Autodesk Inventor part; units mm, degrees
ref_plane "YZ Plane" through (0, 0, 0) normal (1, 0, 0) x (0, 1, 0)
ref_plane "XZ Plane" through (0, 0, 0) normal (0, 1, 0) x (-1, 0, 0)
ref_plane "XY Plane" through (0, 0, 0) normal (0, 0, 1) x (1, 0, 0)
sketch "スケッチ1" plane through (0, 0, 0) normal (1, 0, 0) x (0, 1, 0)
  line L0 (-5, 30) -> (5, 30)
  line L1 (5, 30) -> (5, 0)
  line L2 (5, 0) -> (-5, 0)
  line L3 (-5, 0) -> (-5, 30)
  line L4 (-15, 45) -> (15, 45)
  line L5 (15, 45) -> (15, 30)
  line L6 (15, 30) -> (-15, 30)
  line L7 (-15, 30) -> (-15, 45)
  line L8 (15, 30) -> (5, 0)
  line L9 (-5, 0) -> (-15, 30)
  point P0 (0, 0)
  point P1 (0, 0)
  point P2 (0, 30)
  dimension "d0" = 10
  dimension "d1" = 30
  dimension "d2" = 30
  dimension "d3" = 15
extrude "押し出し1" add sketch "スケッチ1" along normal blind 2
sketch "スケッチ2" plane through (2, 0, 0) normal (1, 0, 0) x (0, 0, -1)
  line L0 (0, -5) -> (0, 5)
  line L1 (-30, 15) -> (-45, 15)
  line L2 (-45, -15) -> (-30, -15)
  point P0 (0, 0)
  point P1 (-37.5, 10)
  point P2 (-37.5, -10)
  point P3 (-25, 0)
  point P4 (-5, 0)
  point P5 (0, 0)
  point P6 (-37.5, 15)
  dimension "d6" = 5
  dimension "d7" = 20
  dimension "d8" = 5
  dimension "d9" = 5
hole "穴1" at (2, 10, 37.5) at (2, -10, 37.5) at (2, 0, 25) at (2, 0, 5) direction (-1, 0, 0) diameter 3.2 end through all
properties part number "FrameJointT1510" material "アルミニウム 6061"
Work out the finished part from the listing and answer in its coordinate system (mm). Give positions to 0.01 mm unless a question says otherwise; leave off trailing zeros. Loops run counter-clockwise (first coordinate to the right, second up) from the corner with the lowest first, then second, coordinate; pieces in that order, holes last. Notation, with made-up numbers: (-32, 1) -> (20, 1) arc R23 cw to (20, 10) -> close; hole circle Ø4 at (13.25, -7.75). An arc over 180 degrees is marked (long way). One line per question, with ' | ' between items. Start each with the question number.
1) Section A-A, the plane y = -10 is taken. Determine the outline of the cut face in (x, z).
2) Straight lines are drawn through the part: L1, parallel to Y at x = 1.15, z = 37.5; L2, parallel to Z at x = 1.2, y = 0; L3, parallel to Z at x = 1, y = -1. For each, find the intervals that lie inside material, in ascending order.
3) Section B-B, the plane z = 5 is taken. Determine the outline of the cut face in (x, y), then the cut area to 3 significant figures.
4) Section C-C, the plane x = 0.5 is taken. Determine the outline of the cut face in (y, z), then the cut area to 3 significant figures.
5) Determine the mould class of faces 1 (the face through (0.99, -1.08, 26.18)), 2 (the face through (1, 0, 0)), 3 (the face through (1, -15, 37)) for opening direction Y: +Y half, -Y half, draft (parallel to the pull), parting line (faces both ways), or undercut.
6) Section D-D, the plane y = -6 is taken. Determine the outline of the cut face in (x, z).
Resolved:
1) outline: (0, 15) -> (2, 15) -> (2, 35.9) -> (0, 35.9) -> close; (0, 39.1) -> (2, 39.1) -> (2, 45) -> (0, 45) -> close
2) L1: -15 to -11.6, -8.4 to 8.4, 11.6 to 15 | L2: 0 to 3.4, 6.6 to 23.4, 26.6 to 45 | L3: 0 to 3.75, 6.25 to 23.75, 26.25 to 45
3) outline: (0, -6.67) -> (2, -6.67) -> (2, -1.6) -> (0, -1.6) -> close; (0, 1.6) -> (2, 1.6) -> (2, 6.67) -> (0, 6.67) -> close | area: 20.3 mm2
4) outline: (-15, 30) -> (-5, 0) -> (5, 0) -> (15, 30) -> (15, 45) -> (-15, 45) -> close; hole circle Ø3.2 at (-10, 37.5); hole circle Ø3.2 at (0, 5); hole circle Ø3.2 at (0, 25); hole circle Ø3.2 at (10, 37.5) | area: 1,020 mm2
5) face 1: undercut | face 2: draft | face 3: -Y half
6) outline: (0, 3) -> (2, 3) -> (2, 45) -> (0, 45) -> close
